For this review, take the finished solid that the model builds, in its own axes (mm). A direction names the side the tool comes from. Coordinates: 2 decimals unless noted, no trailing zeros. Loops run counter-clockwise (first coordinate to the right, second up) from the corner with the lowest first, then second, coordinate; pieces in that order, holes last.
1. Take a section at A-A, the plane z = 4.5. State the section outline as (x, y) points, then the cut area to 3 significant figures.
2. Take a section at B-B, the plane z = 13.25. State the section outline as (x, y) points (3 decimals), then the cut area to 3 significant figures.
3. Machinability: for faces 4 (the face through (-1.2, -1.3, 14)), 5 (the face through (1, -3, 11.5)), 6 (the face through (2, -2, 17.3)), which of the approach directions +Z, -Z, +X, -X, +Y, -Y give a long, thin tool a straight path to every point of the face, cutting with its end or side? Answer none if there is none.
4. Mouldability with a two-part tool opening along X and no side actions: class faces 1 (the face through (-0.635, -4.834, 14.214)), 2 (the face through (0, -1, 7)), 3 (the face through (1, -1, 0)) as pulls with the +X half, pulls with the -X half, needs draft (parallel to the pull), parting line crosses it, or undercut.
5. Clearance check with flat-ended pins moving along their axes: P1, Ø1, axis at y = 1, z = 4, coming from the +X side; P2, Ø3, axis at y = 0.5, z = 16, coming from the +X side (3 decimals); P3, Ø5, axis at x = -1.5, z = 2, coming from the +Y side; P4, Ø1, axis at x = -1.5, z = 10.5, coming from the +Y side. State where each tip first meets the part, or that it passes through.
6. To check wall thickness, follow probe 1 along Y at (x, z) = (0, 5); probe 2 along Z at (x, y) = (1, -3.25); probe 3 along Z at (x, y) = (-1, 2.25). State the ranges of each line that lie inside material, in increasing order.
Autodesk Inventor part; units mm, degrees
ref_plane "YZ Plane" through (0, 0, 0) normal (1, 0, 0) x (0, 1, 0)
ref_plane "XZ Plane" through (0, 0, 0) normal (0, 1, 0) x (-1, 0, 0)
ref_plane "XY Plane" through (0, 0, 0) normal (0, 0, 1) x (1, 0, 0)
sketch "Sketch1" plane through (0, 0, 0) normal (0, 0, 1) x (1, 0, 0)
  circle A0 centre (0, 0) radius 3
  dimension "d0" = 6
extrude "Extrusion1" add sketch "Sketch1" along normal blind 11.5
sketch "Sketch2" plane through (0, 0, 11.5) normal (0, 0, 1) x (1, 0, 0)
  circle A0 centre (0, 0) radius 4.875
  dimension "d3" = 9.75
extrude "Extrusion2" add sketch "Sketch2" along normal blind 5.8
sketch "Sketch3" plane through (0, 0, 17.3) normal (0, 0, 1) x (1, 0, 0)
  line L0 (2.5331, -1.4625) -> (0, -2.925)
  line L1 (0, -2.925) -> (-2.5331, -1.4625)
  line L2 (-2.5331, -1.4625) -> (-2.5331, 1.4625)
  line L3 (-2.5331, 1.4625) -> (0, 2.925)
  line L4 (0, 2.925) -> (2.5331, 1.4625)
  line L5 (2.5331, 1.4625) -> (2.5331, -1.4625)
  point P0 (0, 0)
  point P1 (0, 0)
  point P2 (2.5331, 0)
  dimension "d6" = 5.85
extrude "Extrusion3" cut sketch "Sketch3" against normal blind 3.3
sketch "Sketch4" plane through (0, 0, 14) normal (0, 0, 1) x (1, 0, 0)
  circle A0 centre (0, 0) radius 1
  dimension "d9" = 2
extrude "Extrusion4" cut sketch "Sketch4" against normal through all
chamfer "Chamfer1" distance 0.5 angle 45 1 edges at (-1, 0, 14)
fillet "Fillet1" radius 0.5 1 edges at (-4.875, 0, 17.3)
fillet "Fillet2" radius 0.2 1 edges at (-4.875, 0, 11.5)
thread "Thread1"
chamfer "Chamfer2" distance 0.5 angle 45 1 edges at (-3, 0, 0)
properties part number "fillament guide screw" material "Steel, Alloy"
Results list:
1. outline: circle Ø6 at (0, 0); hole circle Ø2 at (0, 0)
1. area: 25.1 mm2
2. outline: circle Ø9.75 at (0, 0); hole circle Ø2 at (0, 0)
2. area: 71.5 mm2
3. face 4: +Z
3. face 5: -Z
3. face 6: +Z, +X, -X, +Y, -Y
4. face 1: parting line crosses it
4. face 2: undercut
4. face 3: needs draft
5. P1: stops at x = 2.96
5. P2: stops at x = 4.875
5. P3: stops at y = 3
5. P4: stops at y = 2.83
6. probe 1: y = -3 to -1, 1 to 3
6. probe 2: z = 11.5 to 17.3
6. probe 3: z = 0 to 14
